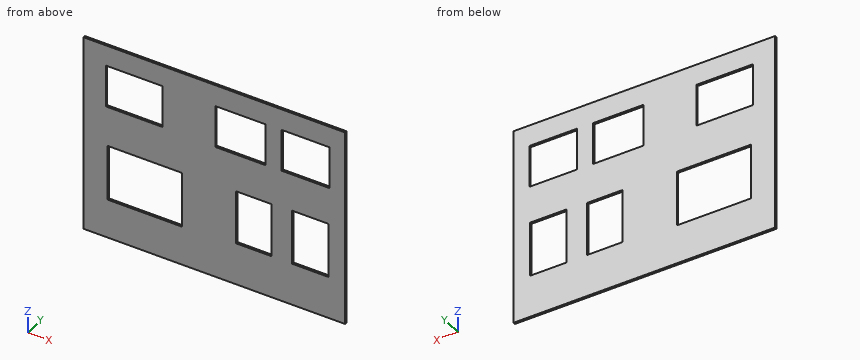
```python
from build123d import *

# Parameters (mm, degrees)
F0_W     = 170.3644944355
F0_H     = 126.3736598194
F0_W_2   = 81.582993269
F0_H_2   = 122.3744936287
F0_W_3   = 83.9825123549
F0_H_3   = 124.7739978135
F0_W_4   = 129.5729912817
F0_H_4   = 95.9800034761
F0_W_5   = 115.175999701
F0_W_6   = 109.5771491528
F1_DEPTH = 5
F2_DEPTH = 5


with BuildPart() as f1:
    # F0 (on Front) → F1 (new body)
    with BuildSketch(Plane.XZ):
        Polygon((362.0641423762, 334.581340097), (-237.9358576238, 334.581340097), (-237.9358576238, 127.1041715145), (-237.9358576238, 87.1041715145), (-237.9358576238, -115.418659903), (362.0641423762, -115.418659903), (362.0641423762, 87.1041715145), (362.0641423762, 109.581340097), (362.0641423762, 127.1041715145), align=None)
        with Locations((-97.5812994875, 36.853896454)):
            Rectangle(F0_W, F0_H, mode=Mode.SUBTRACT)
        with Locations((152.3666083813, 42.0528110117)):
            Rectangle(F0_W_2, F0_H_2, mode=Mode.SUBTRACT)
        with Locations((282.3395207524, 43.252563104)):
            Rectangle(F0_W_3, F0_H_3, mode=Mode.SUBTRACT)
        with Locations((-121.9762098044, 239.211730659)):
            Rectangle(F0_W_4, F0_H_4, mode=Mode.SUBTRACT)
        with Locations((121.9729445875, 237.6120612025)):
            Rectangle(F0_W_5, F0_H_4, mode=Mode.SUBTRACT)
        with Locations((271.1418420076, 238.4118959308)):
            Rectangle(F0_W_6, F0_H_4, mode=Mode.SUBTRACT)
    extrude(amount=F1_DEPTH)

    # F0 (on Front) → F2 (join)
    with BuildSketch(Plane.XZ):
        Polygon((362.0641423762, 334.581340097), (-237.9358576238, 334.581340097), (-237.9358576238, 127.1041715145), (-237.9358576238, 87.1041715145), (-237.9358576238, -115.418659903), (362.0641423762, -115.418659903), (362.0641423762, 87.1041715145), (362.0641423762, 109.581340097), (362.0641423762, 127.1041715145), align=None)
        with Locations((-97.5812994875, 36.853896454)):
            Rectangle(F0_W, F0_H, mode=Mode.SUBTRACT)
        with Locations((152.3666083813, 42.0528110117)):
            Rectangle(F0_W_2, F0_H_2, mode=Mode.SUBTRACT)
        with Locations((282.3395207524, 43.252563104)):
            Rectangle(F0_W_3, F0_H_3, mode=Mode.SUBTRACT)
        with Locations((-121.9762098044, 239.211730659)):
            Rectangle(F0_W_4, F0_H_4, mode=Mode.SUBTRACT)
        with Locations((121.9729445875, 237.6120612025)):
            Rectangle(F0_W_5, F0_H_4, mode=Mode.SUBTRACT)
        with Locations((271.1418420076, 238.4118959308)):
            Rectangle(F0_W_6, F0_H_4, mode=Mode.SUBTRACT)
    extrude(amount=F2_DEPTH)


solid = f1.part
```
Work out the finished part from the listing and answer in its coordinate system (mm). Coordinates: 2 decimals unless noted, no trailing zeros. Loops run counter-clockwise (first coordinate to the right, second up) from the corner with the lowest first, then second, coordinate; pieces in that order, holes last. Notation, with made-up numbers: M 81,61 L 137,61 A37 cw 137,98 Z; hole C 58,-37.5 d10. An arc over 180 degrees is marked long. Use CSV: the item, a comma, the result in double quotes. Start each with the question number.
(1) Find section D-D, the plane x = 300. Give the vertices of the cut face in (y, z), then the cut area to 3 significant figures.
(2) Consider line 1 (Z direction, x = -143.5, y = -4.65); line 2 (Z direction, x = 266, y = -1.45); line 3 (X direction, y = -3.9, z = 268). Determine where each line is inside the solid, lowest interval first.
(3) Find section B-B, the plane z = 232. Give the vertices of the cut face in (x, y).
(4) Find section A-A, the plane x = -68. Give the vertices of the cut face in (y, z), then the cut area to 3 significant figures.
(5) Find section C-C, the plane y = -3.5. Give the vertices of the cut face in (x, z), then the cut area to 3 significant figures.
Recorded:
1,outline,"M -5,-115.42 L 0,-115.42 L 0,-19.13 L -5,-19.13 Z; M -5,105.64 L 0,105.64 L 0,190.42 L -5,190.42 Z; M -5,286.4 L 0,286.4 L 0,334.58 L -5,334.58 Z"
1,area,"1,150 mm^2"
2,line 1,"z = -115.42 to -26.33, 100.04 to 191.22, 287.2 to 334.58"
2,line 2,"z = -115.42 to -19.13, 105.64 to 190.42, 286.4 to 334.58"
2,line 3,"x = -237.94 to -186.76, -57.19 to 64.38, 179.56 to 216.35, 325.93 to 362.06"
3,outline,"M -237.94,-5 L -186.76,-5 L -186.76,0 L -237.94,0 Z; M -57.19,-5 L 64.38,-5 L 64.38,0 L -57.19,0 Z; M 179.56,-5 L 216.35,-5 L 216.35,0 L 179.56,0 Z; M 325.93,-5 L 362.06,-5 L 362.06,0 L 325.93,0 Z"
4,outline,"M -5,-115.42 L 0,-115.42 L 0,-26.33 L -5,-26.33 Z; M -5,100.04 L 0,100.04 L 0,191.22 L -5,191.22 Z; M -5,287.2 L 0,287.2 L 0,334.58 L -5,334.58 Z"
4,area,"1,140 mm^2"
5,outline,"M -237.94,-115.42 L 362.06,-115.42 L 362.06,334.58 L -237.94,334.58 Z; hole M -186.76,191.22 L -57.19,191.22 L -57.19,287.2 L -186.76,287.2 Z; hole M -182.76,-26.33 L -12.4,-26.33 L -12.4,100.04 L -182.76,100.04 Z; hole M 64.38,189.62 L 179.56,189.62 L 179.56,285.6 L 64.38,285.6 Z; hole M 111.58,-19.13 L 193.16,-19.13 L 193.16,103.24 L 111.58,103.24 Z; hole M 216.35,190.42 L 325.93,190.42 L 325.93,286.4 L 216.35,286.4 Z; hole M 240.35,-19.13 L 324.33,-19.13 L 324.33,105.64 L 240.35,105.64 Z"
5,area,"194,000 mm^2"
